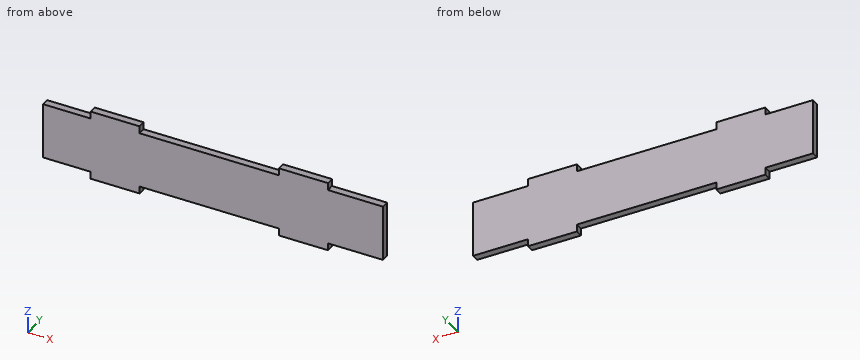
Autodesk Inventor part; units mm, degrees
ref_plane "YZ Plane" through (0, 0, 0) normal (1, 0, 0) x (0, 1, 0)
ref_plane "XZ Plane" through (0, 0, 0) normal (0, 1, 0) x (-1, 0, 0)
ref_plane "XY Plane" through (0, 0, 0) normal (0, 0, 1) x (1, 0, 0)
sketch "Sketch1" plane through (0, 0, 0) normal (0, 1, 0) x (-1, 0, 0)
  line L0 (71, -11.5) -> (-71, -11.5)
  line L1 (-71, -11.5) -> (-71, 11.5)
  line L2 (-71, 11.5) -> (71, 11.5)
  line L3 (71, 11.5) -> (71, -11.5)
  line L4 (68, -11.5) -> (68, 11.5)
  line L5 (48.5, -14.5) -> (28.5, -14.5)
  line L6 (28.5, -14.5) -> (28.5, -11.5)
  line L7 (28.5, -11.5) -> (48.5, -11.5)
  line L8 (48.5, -11.5) -> (48.5, -14.5)
  line L9 (48.5, 11.5) -> (28.5, 11.5)
  line L10 (28.5, 11.5) -> (28.5, 14.5)
  line L11 (28.5, 14.5) -> (48.5, 14.5)
  line L12 (48.5, 14.5) -> (48.5, 11.5)
  line L13 (38.5, -14.5) -> (38.5, -11.5) construction
  line L14 (-48.5, -14.5) -> (-48.5, -11.5)
  line L15 (-38.5, -14.5) -> (-38.5, -11.5) construction
  line L16 (-48.5, -11.5) -> (-28.5, -11.5)
  line L17 (-28.5, 11.5) -> (-48.5, 11.5)
  line L18 (-28.5, -14.5) -> (-48.5, -14.5)
  line L19 (-48.5, 14.5) -> (-28.5, 14.5)
  line L20 (-28.5, 14.5) -> (-28.5, 11.5)
  line L21 (-28.5, -11.5) -> (-28.5, -14.5)
  line L22 (-48.5, 11.5) -> (-48.5, 14.5)
  point P0 (0, 0)
  point P1 (-71, 0)
  point P2 (0, -11.5)
  point P3 (48.5, -11.5)
  point P4 (28.5, -11.5)
  point P5 (-28.5, -11.5)
  point P6 (-48.5, -11.5)
  point P7 (-48.5, 11.5)
  point P8 (-28.5, 11.5)
  point P9 (28.5, 11.5)
  point P10 (48.5, 11.5)
  dimension "d0" = 23
  dimension "d1" = 142
  dimension "d2" = 3
  dimension "d3" = 20
  dimension "d4" = 3
  dimension "d5" = 20
  dimension "d6" = 3
  dimension "d7" = 38.5
  dimension "d10" = 77
extrude "Extrusion1" add sketch "Sketch1" along normal blind 3 contours L0 L1 L2 L4 | L8 L5 L6 L0 | L2 L10 L11 L12 | L21 L18 L14 L0 | L2 L22 L19 L20
equation "\"d0\" = stack"
equation "\"d3\" = finger"
equation "\"d4\" = thickness"
equation "\"d5\" = finger"
equation "\"d15\" = thickness"
equation "\"stack\" = 23"
equation "\"finger\" = 20"
equation "\"thickness\" = 3"
properties part number "BungaSign-Bigger-Sides-LeftRight"
Part model, mm, in its own coordinate system. Coordinates: 2 decimals unless noted, no trailing zeros. Loops run counter-clockwise (first coordinate to the right, second up) from the corner with the lowest first, then second, coordinate; pieces in that order, holes last. Notation, with made-up numbers: M 55.5,50 L 100.5,50 A33 ccw 100.5,89 Z; hole C 55,30 d7. An arc over 180 degrees is marked long. Use a Markdown table: item, result. Add a question column.
Q1. Cut at B-B (x = 0). Write the cut outline in (y, z).
Q2. Probe L1, parallel to Z at x = -0.5, y = 2.95. List the from-to ranges inside material, lowest first.
Q3. Pin check, flat tips, straight feed: P1, Ø0.9, axis at x = 14, y = 1, coming from the -Z side; P2, Ø1.5, axis at y = 1, z = 13.5, coming from the -X side; P3, Ø1.5, axis at y = 1.5, z = 12.5, coming from the +X side. Stop position of each tip, or through.
Q4. Cut at A-A (y = 2.25). Write the cut outline in (x, z).
Worked out:
| question | item | result |
|---|---|---|
| 1 | outline | M 0,-11.5 L 3,-11.5 L 3,11.5 L 0,11.5 Z |
| 2 | L1 | z = -11.5 to 11.5 |
| 3 | P1 | stops at z = -11.5 |
| 3 | P2 | stops at x = -48.5 |
| 3 | P3 | stops at x = 48.5 |
| 4 | outline | M -68,-11.5 L -48.5,-11.5 L -48.5,-14.5 L -28.5,-14.5 L -28.5,-11.5 L 28.5,-11.5 L 28.5,-14.5 L 48.5,-14.5 L 48.5,-11.5 L 71,-11.5 L 71,11.5 L 48.5,11.5 L 48.5,14.5 L 28.5,14.5 L 28.5,11.5 L -28.5,11.5 L -28.5,14.5 L -48.5,14.5 L -48.5,11.5 L -68,11.5 Z |
